Geometry check sheet. Reference: the model listing, model coordinates, mm. Coordinates: 2 decimals unless noted, no trailing zeros. Write each loop counter-clockwise with the first axis right and the second up, starting at its lowest first coordinate (ties: lowest second). Pieces come first, ordered by that corner, then holes. Notation, with made-up numbers: (60, 87) - (89, 87) arc R25 ccw to (89, 124) - close; hole circle Ø8 at (59.5, -1). An arc over 180 degrees is marked (long way). Answer as a JSON object with one key per item and string values. Group by question number.
Autodesk Inventor part; units mm, degrees
ref_plane "YZ Plane" through (0, 0, 0) normal (1, 0, 0) x (0, 1, 0)
ref_plane "XZ Plane" through (0, 0, 0) normal (0, 1, 0) x (-1, 0, 0)
ref_plane "XY Plane" through (0, 0, 0) normal (0, 0, 1) x (1, 0, 0)
ref_plane "Work Plane1" through (0, 0, 0) normal (0, 0, 1) x (1, 0, 0)
sketch "Sketch1" plane through (0, 0, 0) normal (0, 0, 1) x (1, 0, 0)
  circle A0 centre (-0.9133, -5.3891) radius 4
  circle A1 centre (-0.9133, -5.3891) radius 3.8536
  circle A2 centre (-0.9133, -5.3891) radius 5.8
  circle A3 centre (-0.9133, -5.3891) radius 3.2
  point P0 (0, 0)
  dimension "d0" = 1.8
  dimension "d6" = 6.4
extrude "Extrusion1" add sketch "Sketch1" along normal blind 1.6 contours A0 | A1 | A2
chamfer "Chamfer1" distance 0.5 angle 45 2 edges at (-6.7133, -5.3891, 1.6) (-6.7133, -5.3891, 0)
chamfer "Chamfer2" distance 0.5 angle 45 2 edges at (-4.1133, -5.3891, 0) (-4.1133, -5.3891, 1.6)
properties part number "washers"
(1) Draft check along Y on faces 1 (the face through (-1.607, -2.265, 0.796)), 2 (the face through (-5, -6, 1.6)), 3 (the face through (-5.188, -9.309, 0.796)). Enter one of: +Y half, -Y half, draft (parallel to the pull), parting line (faces both ways), or undercut.
(2) Section check A-A (z = 0.25). Record the cut outline in (x, y).
(3) Section check B-B (z = 1.45). Record the cut outline in (x, y).
(4) Material ranges on L1, parallel to X at y = -5.5, z = 0.8; L2, parallel to Y at x = 1.25, z = 0.55; L3, parallel to Y at x = -3.25, z = 0.7, recorded low to high. Write a range as [from, to].
Conclusion:
{
 "1": {"face 1": "undercut", "face 2": "draft", "face 3": "parting line"},
 "2": {"outline": "circle Ø11.1 at (-0.91, -5.39); hole circle Ø6.9 at (-0.91, -5.39)"},
 "3": {"outline": "circle Ø10.9 at (-0.91, -5.39); hole circle Ø7.1 at (-0.91, -5.39)"},
 "4": {"L1": "x = [-6.71, -4.11], [2.28, 4.89]", "L2": "y = [-10.77, -7.75], [-3.03, -0.01]", "L3": "y = [-10.7, -7.58], [-3.2, -0.08]"}
}
